Answer from the drawing. Dimensions are ordinates in mm from the lowest x, y and z of the part. A direction names the side the tool comes from. Give positions to 0.01 mm unless a question says otherwise; leave off trailing zeros. Order: outer loops, then holes, each group sorted by start corner. A loop starts at its lowest first (then second) coordinate and runs counter-clockwise, first axis right, second up. Notation, with made-up numbers: (87, 41.5) - (94, 41.5) arc R22 cw to (94, 62.5) - close; hole circle Ø5 at (28.25, -23.75). An arc over 180 degrees is marked (long way). One line per item, written item: value. Start each with the question number.
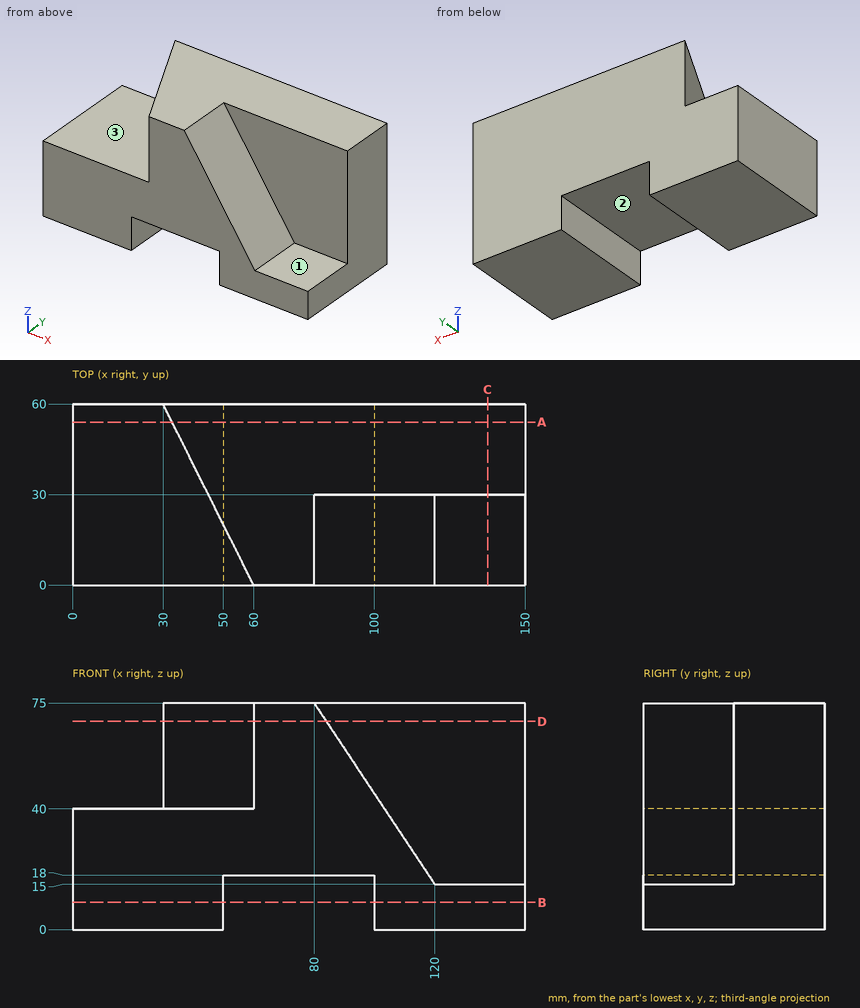
1) Section D-D on z = 69 is taken. Write down the section's boundary in (x, y), plus the area to 3 significant figures.
2) For the marked faces 1, 2 and 3, determine the directions among +Z, -Z, +X, -X, +Y, -Y from which every point of the face is accessible in a straight line to the end or side of a thin tool.
3) Section A-A on y = 54 is taken. Write down the section's boundary in (x, z).
4) Section C-C on x = 137.5 is taken. Write down the section's boundary in (y, z), plus the area to 3 significant figures.
5) Section B-B on z = 9 is taken. Write down the section's boundary in (x, y), plus the area to 3 significant figures.
6) Find the intervals of material crossed by probe 1 along X at (y, z) = (36.5, 5.5); probe 2 along Z at (x, y) = (26.5, 38); probe 3 along Y at (x, z) = (123.5, 71), in increasing order. Write a range as from..to.
7) Each of these flat-tipped pins is pushed along its axis until it touches: pin 1 (8 mm diameter, centred on y = 18.5, z = 20, fed in from +X); pin 2 (4 mm diameter, centred on x = 99, z = 67, fed in from -Y); pin 3 (15 mm diameter, centred on x = 84, y = 15.5, fed in from -Z). Where does it stop, or does it pass through?
Solved:
1. outline: (30, 60) - (60, 0) - (84, 0) - (84, 30) - (150, 30) - (150, 60) - close
1. area: 4,320 mm2
2. face 1: +Z, +X, -Y
2. face 2: -Z, +Y, -Y
2. face 3: +Z, -X, -Y
3. outline: (0, 0) - (50, 0) - (50, 18) - (100, 18) - (100, 0) - (150, 0) - (150, 75) - (33, 75) - (33, 40) - (0, 40) - close
4. outline: (0, 0) - (60, 0) - (60, 75) - (30, 75) - (30, 15) - (0, 15) - close
4. area: 2,700 mm2
5. outline: (0, 0) - (50, 0) - (50, 60) - (0, 60) - close; (100, 0) - (150, 0) - (150, 60) - (100, 60) - close
5. area: 6,000 mm2
6. probe 1: x = 0..50, 100..150
6. probe 2: z = 0..40
6. probe 3: y = 30..60
7. pin 1: stops at x = 119.33
7. pin 2: stops at y = 30
7. pin 3: stops at z = 18
